Autodesk Inventor part; units mm, degrees
ref_plane "YZ Plane" through (0, 0, 0) normal (1, 0, 0) x (0, 1, 0)
ref_plane "XZ Plane" through (0, 0, 0) normal (0, 1, 0) x (-1, 0, 0)
ref_plane "XY Plane" through (0, 0, 0) normal (0, 0, 1) x (1, 0, 0)
ref_plane "Plano de trabajo1" through (0, 0, 0) normal (0, 0, 1) x (1, 0, 0)
sketch "Boceto1" plane through (0, 0, 0) normal (0, 0, 1) x (1, 0, 0)
  circle A0 centre (10.9923, 0) radius 10.9823
  circle A1 centre (10.9923, 0) radius 3.1378
  circle A2 centre (18.3423, 0) radius 1.2028
  circle A3 centre (10.9923, 7.35) radius 1.2028
  circle A4 centre (3.6423, 0) radius 1.2028
  circle A5 centre (10.9923, -7.35) radius 1.2028
  line L0 (0, 0) -> (0, 30)
  line L1 (21.9746, 0) -> (21.9746, -30)
  line L2 (0, 0) -> (0, -30)
  line L3 (0, -30) -> (21.9746, -30)
  circle A6 centre (10.9923, 0) radius 3.1378
  circle A7 centre (18.3423, 0) radius 1.2028
  circle A8 centre (10.9923, -7.35) radius 1.2028
  circle A9 centre (3.6423, 0) radius 1.2028
  circle A10 centre (10.9923, 7.35) radius 1.2028
  circle A11 centre (10.9923, 0) radius 10.9823
  line L4 (0, 0) -> (0, -30)
  line L5 (0, -30) -> (21.9746, -30)
  line L6 (21.9746, -30) -> (21.9746, 0)
  dimension "d0" = 30
  dimension "d1" = 30
extrude "Extrusión1" add sketch "Boceto1" along normal blind 3
sketch "Boceto2" plane through (10.9923, 0, 3) normal (0, 0, 1) x (1, 0, 0)
  circle A0 centre (0, 0) radius 10.9823
  line L0 (10.9823, 0) -> (10.9823, -30)
  line L1 (10.9823, -30) -> (-9.7118, -30)
  line L2 (-9.7118, -30) -> (-10.9923, 0)
  circle A1 centre (0, 0) radius 10.9823
  circle A2 centre (0, -7.35) radius 1.2028
  circle A3 centre (-7.35, 0) radius 1.2028
  circle A4 centre (0, 7.35) radius 1.2028
  circle A5 centre (7.35, 0) radius 1.2028
  circle A6 centre (0, 0) radius 3.1378
  point P0 (-10.9723, -0.4683)
  dimension "d4" = 30
extrude "Extrusión2" add sketch "Boceto2" against normal blind 3 contours L0 L1 L2 A0
sketch "Boceto3" plane through (0, 0, 0) normal (0, 0, -1) x (-1, 0, 0)
  point P0 (0, 0)
sketch "Boceto4" plane through (0, 0, 3) normal (0, 0, 1) x (1, 0, 0)
  point P0 (0, 0)
sketch "Boceto5" plane through (0, 0, 0) normal (0, 0, -1) x (-1, 0, 0)
  arc A0 (-0.02, -0.4683) -> (-21.9746, 0) centre (-10.9923, 0) ccw
  line L0 (-21.9746, 0) -> (-21.9746, -30)
  line L1 (-21.9746, -30) -> (-1.2805, -30)
  line L2 (-1.2805, -30) -> (-0.02, -0.4683)
  circle A1 centre (-10.9923, -7.35) radius 1.2028
  circle A2 centre (-3.6423, 0) radius 1.2028
  circle A3 centre (-10.9923, 7.35) radius 1.2028
  circle A4 centre (-18.3423, 0) radius 1.2028
  circle A5 centre (-10.9923, 0) radius 3.1378
  line L3 (-21.9746, -30) -> (0, -30)
  line L4 (0, -30) -> (0, 0)
  line L5 (0, 0) -> (-21.9746, 0)
  line L6 (-21.9746, 0) -> (-21.9746, -30)
  point P0 (-0.01, 0)
extrude "Extrusión3" add sketch "Boceto5" against normal blind 3 contours A0 L5 L4 L3 L2
sketch "Boceto6" plane through (0, 0, 0) normal (0, 0, -1) x (-1, 0, 0)
  point P0 (0, 0)
sketch "Boceto7" plane through (0, 0, 0) normal (0, 0, -1) x (-1, 0, 0)
  line L0 (-21.9746, -30) -> (0, -30)
  line L1 (-21.9746, -30) -> (-21.9746, 0)
  line L2 (0, -30) -> (-21.9746, -30)
  line L3 (-21.9746, -30) -> (-21.9746, -27)
  line L4 (-21.9746, -27) -> (0, -27)
  line L5 (0, -27) -> (0, -30)
  point P0 (0, 0)
  dimension "d9" = 3
extrude "Extrusión4" add sketch "Boceto7" along normal blind 40
sketch "Boceto8" plane through (0, -27, 0) normal (0, 1, 0) x (1, 0, 0)
  line L0 (0, -3) -> (0, 40)
  line L1 (21.9746, -3) -> (21.9746, 40)
  line L2 (0, 40) -> (21.9746, 40)
  line L3 (21.9746, 40) -> (21.9746, 38)
  line L4 (21.9746, 38) -> (0, 38)
  line L5 (0, 38) -> (0, 40)
  point P0 (0, 0)
  point P1 (21.9746, 40)
  point P2 (0, 38)
  dimension "d12" = 2
extrude "Extrusión5" add sketch "Boceto8" along normal blind 40
sketch "Boceto9" plane through (0, 0, -40) normal (0, 0, -1) x (-1, 0, 0)
  circle A0 centre (-11.0072, -0.015) radius 2.7
  circle A1 centre (-11.0072, -0.015) radius 10.9823
  circle A2 centre (-18.3423, 0) radius 1.2028
  circle A3 centre (-10.9923, -7.35) radius 1.2028
  circle A4 centre (-10.9923, 7.35) radius 1.2028
  circle A5 centre (-3.6423, 0) radius 1.2028
  line L0 (-21.9746, -30) -> (-21.9746, 13)
  line L1 (-21.9746, -30) -> (0, -30)
  line L2 (0, -30) -> (0, 13)
  line L3 (-21.9746, 13) -> (0, 13)
  line L4 (-21.5706, 0) -> (-25.972, 0)
  line L5 (-25.972, 0) -> (-25.972, 18.1609)
  line L6 (-25.972, 18.1609) -> (4.5124, 18.1609)
  line L7 (4.5124, 18.1609) -> (4.5124, 1.2028)
  line L8 (4.5124, 1.2028) -> (4.5124, 0)
  line L9 (-3.6423, 0) -> (4.822, 0)
  point P0 (0, 0)
  point P1 (-21.9746, 0.557)
  point P2 (-0.0249, 0)
  point P3 (0, 0)
extrude "Extrusión6" cut sketch "Boceto9" against normal blind 40 contours A0 | A1 L0 L3 L2 L9 | A2 | A3 | A4 | A5
sketch "Boceto10" plane through (0, -30, 3) normal (0, -1, 0) x (1, 0, 0)
  point P0 (0, -3)
sketch "Boceto11" plane through (0, -30, 3) normal (0, -1, 0) x (1, 0, 0)
  line L0 (0.0249, -43) -> (21.9746, -43)
  line L1 (0, -3) -> (0, 0)
  line L2 (21.9746, -43) -> (0, -43)
  line L3 (0, -43) -> (0, 0)
  line L4 (0, 0) -> (21.9746, 0)
  line L5 (21.9746, 0) -> (21.9746, -43)
  line L6 (0, -43) -> (-100, -43)
  line L7 (-100, -43) -> (-100, 0)
  line L8 (-100, 0) -> (0, 0)
  line L9 (0, 0) -> (0, -43)
  line L10 (-100, 0) -> (-100, -21.5)
  line L11 (-100, -21.5) -> (-100, -14.5)
  line L12 (-100, -14.5) -> (-100, -28.5)
  line L13 (-100, -28.5) -> (-50, -43)
  line L14 (-50, -43) -> (-50, 0)
  line L15 (-100, -14.5) -> (-50, 0)
  dimension "d17" = 100
  dimension "d18" = 21.5
  dimension "d19" = 7
  dimension "d20" = 14
extrude "Extrusión7" add sketch "Boceto11" along normal blind 10 contours L2 L3 L1 L4 L5 L0 | L6 L14 L8 L1 L3 | L13 L7 L15 L14
chamfer "Chaflán1" distance 2 angle 45 12 edges at (-14.0127, -40, -40) (-75, -40, -32.75) (-75, -30, -32.75) (-25, -30, -40) (-14.0127, -40, 3) (-75, -40, -4.25) (-100, -40, -18.5) (-75, -30, -4.25) (-25, -30, 3) (-100, -30, -18.5) (-100, -35, -25.5) (-100, -35, -11.5)
sketch "Boceto12" plane through (0, -40, 3) normal (0, -1, 0) x (1, 0, 0)
  line L0 (-49.7159, -2) -> (21.9746, -2)
  line L1 (-98, -16.0024) -> (-49.7159, -2)
  line L2 (-98, -26.9976) -> (-98, -16.0024)
  line L3 (-49.7159, -41) -> (-98, -26.9976)
  line L4 (21.9746, -41) -> (-49.7159, -41)
  line L5 (21.9746, -41) -> (21.9746, -2)
  line L6 (-48.5793, -33) -> (-88.2344, -21.5)
  line L7 (-88.2344, -21.5) -> (-48.5793, -10)
  line L8 (-48.5793, -10) -> (13.9746, -10)
  line L9 (13.9746, -10) -> (13.9746, -33)
  line L10 (13.9746, -33) -> (-48.5793, -33)
  point P0 (0, -3)
  dimension "d26" = 8
extrude "Extrusión8" cut sketch "Boceto12" against normal blind 4 contours L6 L7 L8 L9 L10
properties part number "tibia"
Geometry check sheet. Reference: the model listing, model coordinates, mm. A direction names the side the tool comes from. Round coordinates to 2 decimals unless told otherwise and drop trailing zeros. Loops run counter-clockwise (first coordinate to the right, second up) from the corner with the lowest first, then second, coordinate; pieces in that order, holes last.
Item 1: Cross-section at A-A on y = -7.35. Record the boundary of the cut face in (x, z), then the cut area to 3 significant figures.
Item 2: Mould release check, pull along Y, two halves, no side actions. Record for faces 5 (the cylindrical face through (9.88, -7.81, -39.01)), 6 (the flat face through (-74, -31, -32)), 7 (the flat face through (21.975, -29, -13)): pulls with the +Y half, pulls with the -Y half, needs draft (parallel to the pull), parting line crosses it, or undercut.
Item 3: Thickness scan on line 1 (Z direction, x = 14, y = -6); line 2 (Y direction, x = 8.5, z = -5); line 3 (Y direction, x = -45, z = -32). Record the ranges inside material, lowest first.
Item 4: Cross-section at B-B on x = -46.5. Record the boundary of the cut face in (y, z), then the cut area to 3 significant figures.
Item 5: Cross-section at D-D on x = -70. Record the boundary of the cut face in (y, z).
Item 6: Access from +Z, -Z, +X, -X, +Y, -Y to the whole of each face (thin tool, end or side, straight path). Record for faces 1 (the flat face through (11, -27, -19)), 2 (the cylindrical face through (12.103, 7.811, 1.479)), 3 (the flat face through (-68.13, -38.03, -24.33)), 4 (the flat face through (-39, -30, -18)).
Item 7: Gauge pin test, flat ends, axial feed: pin 1 (1.2 mm diameter, centred on y = -39, z = -18.5, fed in from -X); pin 2 (1.4 mm diameter, centred on x = 10.99, y = 7.35, fed in from +Z); pin 3 (12 mm diameter, centred on x = -43, z = -2, fed in from +Y); pin 4 (18.5 mm diameter, centred on x = -38, z = -19, fed in from -Y). Record the tip position at first contact, or that the pin passes through.
Item 8: Cross-section at C-C on y = 7.35. Record the boundary of the cut face in (x, z), then the cut area to 3 significant figures.
Answer sheet:
1. outline: (0, -40) - (9.79, -40) - (9.79, -38) - (0, -38) - close; (0, 0) - (9.79, 0) - (9.79, 3) - (0, 3) - close; (12.2, -40) - (21.97, -40) - (21.97, -38) - (12.2, -38) - close; (12.2, 0) - (21.97, 0) - (21.97, 3) - (12.2, 3) - close
1. area: 97.8 mm2
2. face 5: undercut
2. face 6: pulls with the +Y half
2. face 7: needs draft
3. line 1: z = -40 to -38, 0 to 3
3. line 2: y = -40 to -27
3. line 3: y = -40 to -30
4. outline: (-40, -38) - (-38, -40) - (-32, -40) - (-30, -38) - (-30, 1) - (-32, 3) - (-38, 3) - (-40, 1) - (-40, -7) - (-36, -7) - (-36, -30) - (-40, -30) - close
4. area: 330 mm2
5. outline: (-40, -32.12) - (-38, -34.2) - (-32, -34.2) - (-30, -32.12) - (-30, -4.88) - (-32, -2.8) - (-38, -2.8) - (-40, -4.88) - (-40, -13.21) - (-36, -13.21) - (-36, -23.79) - (-40, -23.79) - close
6. face 1: +X, -X, +Y
6. face 2: +Z, -Z
6. face 3: -Y
6. face 4: +Z, -Z, -X, +Y
7. pin 1: stops at x = -99.6
7. pin 2: passes through
7. pin 3: stops at y = -30
7. pin 4: stops at y = -36
8. outline: (2.83, 0) - (9.79, 0) - (9.79, 3) - (2.83, 3) - close; (2.86, -40) - (9.79, -40) - (9.79, -38) - (2.86, -38) - close; (12.2, -40) - (19.15, -40) - (19.15, -38) - (12.2, -38) - close; (12.2, 0) - (19.15, 0) - (19.15, 3) - (12.2, 3) - close
8. area: 69.5 mm2
